Verification items for the finished model (mm, model axes). A direction names the side the tool comes from. Round coordinates to 2 decimals unless told otherwise and drop trailing zeros. Order: outer loops, then holes, each group sorted by start corner. A loop starts at its lowest first (then second) coordinate and runs counter-clockwise, first axis right, second up. Notation, with made-up numbers: (-40, 69) -> (-30, 69) arc R23 cw to (-30, 98) -> close; hole circle Ø9 at (21.25, 10.5). An arc over 180 degrees is marked (long way). Return JSON: item names as keys, results as strings. Group by question number.
1) Tool access check on faces 1 (the flat face through (-9.25, 2.27, -3.84)), 2 (the flat face through (-8, 2, 1.05)), 3 (the flat face through (-55, 2, -10.825)). Record the directions out of +Z, -Z, +X, -X, +Y, -Y that give a thin tool (end or side, any length) a straight path to the whole face; none if there is none.
2) Section check C-C on x = -45.5. Enter the section's corners in (y, z), plus the area to 4 significant figures.
3) Section check A-A on y = 2.3. State how many separate pieces and enclosed holes the cut face has, plus the area to 3 significant figures.
4) Draft check along Z on faces 4 (the flat face through (-52.675, 3, -8)), 5 (the cylindrical face through (-54.65, 1.92, 6.1)), 6 (the flat face through (7.893, 2.268, -3.81)). Enter one of: pulls with the +Z half, pulls with the -Z half, needs draft (parallel to the pull), parting line crosses it, or undercut.
5) Depth check by flat-ended pin: pin 1 (1.4 mm diameter, centred on x = 31.5, y = 3.5, fed in from -Z); pin 2 (0.7 mm diameter, centred on x = 7, y = 2.5, fed in from -Z); pin 3 (2 mm diameter, centred on y = 1, z = 4, fed in from +X). Enter the tip coordinate at first touch or a pass-through.
6) Scan lines: L1, parallel to Z at x = -31, y = 0.4; L2, parallel to X at y = 2.5, z = -8.25; L3, parallel to Z at x = 23, y = 3.2. Record each from-to range of solid material in increasing order.
7) Section check B-B on z = -9. Enter the section's corners in (x, y), plus the area to 3 significant figures.
```python
from build123d import *

# Parameters (mm, degrees)
BOSS_EXTRUDE1_DEPTH  = 4.6
SKETCH11_W           = 3.75
SKETCH11_H           = 4.6
BOSS_EXTRUDE14_DEPTH = 30
SKETCH18_W           = 20
SKETCH18_H           = 4.6
SKETCH18_R           = 1
BOSS_EXTRUDE15_DEPTH = 4
SKETCH19_W           = 3.75
SKETCH19_H           = 4.6
BOSS_EXTRUDE16_DEPTH = 10


with BuildPart() as part:
    # Sketch1 → Boss-Extrude1 (new body)
    with BuildSketch(Plane(origin=(0, 0, 0), x_dir=(1, 0, 0), z_dir=(0, 1, 0))):
        Polygon((27.324900936, 2.700375145), (27.145947966, 2.700375145), (26.327014939, 4.950375145), (25.712159083, 4.950375145), (24.893226056, 2.700375145), (24.004355316, 2.700375145), (23.185422289, 4.950375145), (22.570566433, 4.950375145), (21.751633406, 2.700375145), (20.862762666, 2.700375145), (20.043829639, 4.950375145), (19.428973783, 4.950375145), (18.610040756, 2.700375145), (17.721170016, 2.700375145), (16.902236989, 4.950375145), (16.287381133, 4.950375145), (15.468448106, 2.700375145), (14.579577366, 2.700375145), (13.760644339, 4.950375145), (13.145788483, 4.950375145), (12.326855456, 2.700375145), (11.437984716, 2.700375145), (10.619051689, 4.950375145), (10.004195833, 4.950375145), (9.185262806, 2.700375145), (8.296392066, 2.700375145), (7.477459039, 4.950375145), (6.862603183, 4.950375145), (6.043670156, 2.700375145), (5.154799416, 2.700375145), (4.335866389, 4.950375145), (3.721010533, 4.950375145), (2.902077506, 2.700375145), (2.013206766, 2.700375145), (1.194273739, 4.950375145), (0.579417883, 4.950375145), (-0.239515144, 2.700375145), (-1.128385884, 2.700375145), (-1.947318911, 4.950375145), (-2.562174767, 4.950375145), (-3.381107794, 2.700375145), (-4.269978534, 2.700375145), (-5.088911561, 4.950375145), (-5.703767417, 4.950375145), (-6.522700444, 2.700375145), (-7.411571184, 2.700375145), (-8.230504211, 4.950375145), (-8.845360067, 4.950375145), (-9.664293094, 2.700375145), (-10.553163834, 2.700375145), (-11.372096861, 4.950375145), (-11.986952717, 4.950375145), (-12.805885744, 2.700375145), (-13.694756484, 2.700375145), (-14.513689511, 4.950375145), (-15.128545367, 4.950375145), (-15.947478394, 2.700375145), (-16.836349134, 2.700375145), (-17.655282161, 4.950375145), (-18.270138017, 4.950375145), (-19.089071044, 2.700375145), (-19.977941784, 2.700375145), (-20.796874811, 4.950375145), (-21.411730667, 4.950375145), (-22.230663694, 2.700375145), (-22.675099064, 2.700375145), (-22.675099064, -1.049624855), (27.324900936, -1.049624855), align=None)
    extrude(amount=BOSS_EXTRUDE1_DEPTH)

    # Sketch11 → Boss-Extrude14 (add)
    with BuildSketch(Plane.ZY.offset(22.675099064)):
        with Locations((-0.825375145, 2.3)):
            Rectangle(SKETCH11_W, SKETCH11_H)
    extrude(amount=BOSS_EXTRUDE14_DEPTH)

    # Sketch18 → Boss-Extrude15 (add)
    with BuildSketch(Plane.ZY.offset(52.675099064)):
        with Locations((-0.825375145, 2.3)):
            Rectangle(SKETCH18_W, SKETCH18_H)
        with Locations((5.174624855, 2.3)):
            Circle(SKETCH18_R, mode=Mode.SUBTRACT)
        with Locations((-6.825375145, 2.3)):
            Circle(SKETCH18_R, mode=Mode.SUBTRACT)
    extrude(amount=BOSS_EXTRUDE15_DEPTH)

    # Sketch19 → Boss-Extrude16 (add)
    with BuildSketch(Plane(origin=(27.324900936, 0, 0), x_dir=(0, 0, -1), z_dir=(1, 0, 0))):
        with Locations((0.825375145, 2.3)):
            Rectangle(SKETCH19_W, SKETCH19_H)
    extrude(amount=BOSS_EXTRUDE16_DEPTH)


solid = part.part
```
Check result:
{
 "1": {"face 1": "-Z, +Y, -Y", "face 2": "+Z, +X, +Y, -Y", "face 3": "-Z, +X, -X, +Y, -Y"},
 "2": {"outline": "(0, -2.7) -> (4.6, -2.7) -> (4.6, 1.05) -> (0, 1.05) -> close", "area": "17.25 mm^2"},
 "3": {"separate pieces": "3", "enclosed holes": "0", "area": "453 mm^2"},
 "4": {"face 4": "needs draft", "face 5": "undercut", "face 6": "pulls with the -Z half"},
 "5": {"pin 1": "z = -2.7", "pin 2": "z = -4.95", "pin 3": "x = -52.68"},
 "6": {"L1": "-2.7 to 1.05", "L2": "-56.68 to -52.68", "L3": "-4.95 to 1.05"},
 "7": {"outline": "(-56.68, 0) -> (-52.68, 0) -> (-52.68, 4.6) -> (-56.68, 4.6) -> close", "area": "18.4 mm^2"}
}
